Can you work these out from the model? Positions are in its coordinate system, mm. A direction names the side the tool comes from. Give positions to 0.01 mm unless a question says otherwise; leave off trailing zeros. Order: outer loops, then holes, each group sorted by start corner. A loop starts at its lowest first (then second) coordinate and runs counter-clockwise, first axis right, second up. Notation, with made-up numbers: (-2, 54) - (10, 54) arc R12 ccw to (10, 75) - close; hole circle Ø5 at (-22.75, 69). An arc over 180 degrees is marked (long way). Use one line per item in the form item = value. Start each with the question number.
1) Suppose I cut it at D-D, the plane x = 9. Write out the boundary of the cut face in (y, z).
2) Please list where these lines run through material, in increasing order: probe 1 along X at (y, z) = (23.25, -17.75); probe 2 along Z at (x, y) = (13.25, 23.75); probe 3 along X at (y, z) = (4, -15.75).
3) Suppose I cut it at B-B, the plane z = -28. Write out the boundary of the cut face in (x, y), and give its area (3 significant figures).
4) We'd pull the mould along X, two halves only. Please class faces 1 (the flat face through (8, 17, -5.5)), 2 (the flat face through (0.5, 10, -19)), 3 (the flat face through (3, 27, -8)): released by +X, released by -X, zero draft, split by the parting line, or undercut.
5) Suppose I cut it at A-A, the plane y = 25. Write out the boundary of the cut face in (x, z).
6) Which directions (+Z, -Z, +X, -X, +Y, -Y) give clear straight access to the entire face, cutting with the end or side of a thin tool? Please do faces 4 (the flat face through (14, 1, -15)), 5 (the cylindrical face through (3.01, 8.11, -16.02)), 6 (the flat face through (0, 17, -11)).
7) Suppose I cut it at C-C, the plane y = 12.5. Write out the boundary of the cut face in (x, z).
8) For pin 1 (8 mm diameter, centred on y = 12, z = -11, fed in from -X); pin 2 (8 mm diameter, centred on y = 12.5, z = -15.1, fed in from -X); pin 3 (0.8 mm diameter, centred on x = 2.5, z = -11, fed in from +Y); pin 4 (7.5 mm diameter, centred on x = 13, z = -11, fed in from +Y), each with a flat end and sliding along its axis, tell me the tip position at first contact or that it passes through.
```python
from build123d import *

# Parameters (mm, degrees)
SKETCH2_W           = 30
SKETCH2_H           = 27
BOSS_EXTRUDE1_DEPTH = 20
SKETCH6_W           = 7
SKETCH6_H           = 27
CUT_EXTRUDE4_DEPTH  = 26
SKETCH9_W           = 6
SKETCH9_H           = 16
CUT_EXTRUDE5_DEPTH  = 21
SKETCH11_R          = 5
CUT_EXTRUDE8_DEPTH  = 0.5
SKETCH12_W          = 2.75
SKETCH12_H          = 12
CUT_EXTRUDE12_DEPTH = 17.5
SKETCH15_R          = 4.5
CUT_EXTRUDE13_DEPTH = 5


with BuildPart() as part:
    # Sketch2 → Boss-Extrude1 (new body)
    with BuildSketch(Plane(origin=(0, 0, 0), x_dir=(0, 0, -1), z_dir=(1, 0, 0))):
        with Locations((15, 13.5)):
            Rectangle(SKETCH2_W, SKETCH2_H)
    extrude(amount=BOSS_EXTRUDE1_DEPTH)

    # Sketch6 → Cut-Extrude4 (cut)
    with BuildSketch(Plane(origin=(2.296116437, 27, -0.293484995), x_dir=(1, 0, 0), z_dir=(0, 1, 0))):
        with Locations((11.865844825, 14.706515005)):
            Rectangle(SKETCH6_W, SKETCH6_H)
    extrude(amount=-CUT_EXTRUDE4_DEPTH, mode=Mode.SUBTRACT)

    # Sketch9 → Cut-Extrude5 (cut)
    with BuildSketch(Plane(origin=(0, 27, 0), x_dir=(1, 0, 0), z_dir=(0, 1, 0))):
        with Locations((7.661961261, 13.5)):
            Rectangle(SKETCH9_W, SKETCH9_H)
    extrude(amount=-CUT_EXTRUDE5_DEPTH, mode=Mode.SUBTRACT)

    # Sketch11 → Cut-Extrude8 (cut)
    with BuildSketch(Plane.ZY):
        with Locations((-15.1, 12.5)):
            Circle(SKETCH11_R)
    extrude(amount=-CUT_EXTRUDE8_DEPTH, mode=Mode.SUBTRACT)

    # Sketch12 → Cut-Extrude12 (cut)
    with BuildSketch(Plane(origin=(0, 27, 0), x_dir=(1, 0, 0), z_dir=(0, 1, 0))):
        with Locations((2.286961261, 15)):
            Rectangle(SKETCH12_W, SKETCH12_H)
    extrude(amount=-CUT_EXTRUDE12_DEPTH, mode=Mode.SUBTRACT)

    # Sketch15 → Cut-Extrude13 (cut)
    with BuildSketch(Plane.ZY.offset(-0.5)):
        with Locations((-15.04, 12.5)):
            Circle(SKETCH15_R)
    extrude(amount=-CUT_EXTRUDE13_DEPTH, mode=Mode.SUBTRACT)


solid = part.part
```
Result sheet:
q1.outline = (0, -30) - (27, -30) - (27, -21.5) - (6, -21.5) - (6, -5.5) - (27, -5.5) - (27, 0) - (0, 0) - close
q2.probe_1 = 0 to 0.91, 3.66 to 4.66, 17.66 to 20
q2.probe_2 = -30 to -28.5, -1.5 to 0
q2.probe_3 = 0 to 10.66, 17.66 to 20
q3.outline = (0, 0) - (20, 0) - (20, 27) - (17.66, 27) - (17.66, 1) - (10.66, 1) - (10.66, 27) - (0, 27) - close
q3.area = 358 mm²
q4.face_1 = undercut
q4.face_2 = released by -X
q4.face_3 = zero draft
q5.outline = (0, -30) - (20, -30) - (20, 0) - (0, 0) - close; hole (0.91, -21) - (3.66, -21) - (3.66, -9) - (0.91, -9) - close; hole (4.66, -21.5) - (10.66, -21.5) - (10.66, -28.5) - (17.66, -28.5) - (17.66, -1.5) - (10.66, -1.5) - (10.66, -5.5) - (4.66, -5.5) - close
q6.face_4 = +Y
q6.face_5 = -X
q6.face_6 = +Z, -Z, -X, +Y, -Y
q7.outline = (0, -30) - (20, -30) - (20, 0) - (0, 0) - (0, -10.1) - (0.5, -10.1) - (0.5, -10.54) - (0.91, -10.54) - (0.91, -9) - (3.66, -9) - (3.66, -10.54) - (4.66, -10.54) - (4.66, -5.5) - (10.66, -5.5) - (10.66, -1.5) - (17.66, -1.5) - (17.66, -28.5) - (10.66, -28.5) - (10.66, -21.5) - (4.66, -21.5) - (4.66, -19.54) - (3.66, -19.54) - (3.66, -21) - (0.91, -21) - (0.91, -19.54) - (0.5, -19.54) - (0.5, -20.1) - (0, -20.1) - close
q8.pin_1 = 0
q8.pin_2 = 17.66
q8.pin_3 = 9.5
q8.pin_4 = 6
